Work out the finished part from the listing and answer in its coordinate system (mm). Give positions to 0.01 mm unless a question says otherwise; leave off trailing zeros. Write each loop counter-clockwise with the first axis right and the second up, starting at its lowest first coordinate (ties: lowest second). Pieces come first, ordered by that corner, then holes.
1) Find section B-B (y = 132.5). Determine the outline of the cut face in (x, z).
2) Find section D-D (x = 178.5). Determine the outline of the cut face in (y, z).
3) Straight lines are drawn through the part: probe 1 along X at (y, z) = (11, 1.5); probe 2 along Z at (x, y) = (-214.5, 116); probe 3 along X at (y, z) = (8, 2.75). For each, find the intervals that lie inside material, in ascending order.
4) Find section C-C (y = -32.5). Count the separate pieces of the cut face and the enclosed holes in it, plus the area to 3 significant figures.
5) Determine the mould class of faces 1 (the face through (-174.115, -38.296, 3.042)), 2 (the face through (-2.62, -41.8, 3.04)), 3 (the face through (-203, -32, 8)) for opening direction Y: pulls with the +Y half, pulls with the -Y half, needs draft (parallel to the pull), parting line crosses it, or undercut.
6) Given pin 1 Ø0.6 at (y, z) = (-25.5, 6.5) entering from -X; pin 2 Ø0.6 at (y, z) = (5.5, 6.5) entering from +X; pin 3 Ø0.6 at (x, z) = (-120, 6.5) entering from -Y, each flat-ended and moving along its own axis, determine where each tip first touches the part or whether it passes through.
7) Find section A-A (x = -204). Determine the outline of the cut face in (y, z), plus the area to 3 significant figures.
```python
from build123d import *

# Parameters (mm, degrees)
ESBO_O1_W                 = 485
ESBO_O1_H                 = 450
RESSALTO_EXTRUS_O1_DEPTH  = 6
ESBO_O2_W                 = 39.943598922
ESBO_O2_H                 = 30
RESSALTO_EXTRUS_O2_DEPTH  = 2
PADR_O_LINEAR1_COUNT      = 4
PADR_O_LINEAR1_PITCH      = 83
PADR_O_LINEAR1_COUNT_DIR2 = 2
PADR_O_LINEAR1_PITCH_DIR2 = 40
ESBO_O3_R                 = 9.525
CORTE_EXTRUS_O1_DEPTH     = 331.858353378
PADR_O_LINEAR2_COUNT      = 4
PADR_O_LINEAR2_PITCH      = 83
PADR_O_LINEAR2_COUNT_DIR2 = 2
PADR_O_LINEAR2_PITCH_DIR2 = 40
CHANFRO1_SIZE             = 2
CHANFRO1_SIZE2            = 3.464101615


with BuildPart() as part:
    # Esboço1 → Ressalto-extrusão1 (new body)
    with BuildSketch(Plane.XY):
        Rectangle(ESBO_O1_W, ESBO_O1_H)
    extrude(amount=RESSALTO_EXTRUS_O1_DEPTH)

    # Esboço2 → Ressalto-extrusão2 (add)
    with BuildSketch(Plane.XY.offset(6)):
        with Locations((-202.528200539, 7.5)):
            Rectangle(ESBO_O2_W, ESBO_O2_H)
    ressalto_extrus_o2 = extrude(amount=RESSALTO_EXTRUS_O2_DEPTH)

    # Padrão linear1: Ressalto-extrus_o2 4 × 2
    with Locations(*[(i * PADR_O_LINEAR1_PITCH, -j * PADR_O_LINEAR1_PITCH_DIR2, 0) for i in range(PADR_O_LINEAR1_COUNT) for j in range(PADR_O_LINEAR1_COUNT_DIR2) if (i, j) != (0, 0)]):
        add(ressalto_extrus_o2)

    # Esboço3 → Corte-extrusão1 (cut, through all)
    with BuildSketch(Plane.XY.offset(6)):
        with Locations((-166.556401078, 7.5)):
            Circle(ESBO_O3_R)
    corte_extrus_o1 = extrude(amount=-CORTE_EXTRUS_O1_DEPTH, mode=Mode.SUBTRACT)

    # Padrão linear2: Corte-extrus_o1 4 × 2
    with Locations(*[(i * PADR_O_LINEAR2_PITCH, -j * PADR_O_LINEAR2_PITCH_DIR2, 0) for i in range(PADR_O_LINEAR2_COUNT) for j in range(PADR_O_LINEAR2_COUNT_DIR2) if (i, j) != (0, 0)]):
        add(corte_extrus_o1, mode=Mode.SUBTRACT)

    # Chanfro1
    chanfro1_edges = [part.edges().sort_by_distance(p)[0] for p in [
        (0, 225, 0),
        (242.5, 0, 0),
        (0, -225, 0),
        (-242.5, 0, 0),
    ]]
    chanfro1_side = [part.faces().sort_by_distance(p)[0] for p in [
        (0, -218.383921101, 0),
    ]]
    chamfer(chanfro1_edges, length=CHANFRO1_SIZE, length2=CHANFRO1_SIZE2, reference=chanfro1_side[0])


solid = part.part
```
Results:
1. outline: (-242.5, 3.46) - (-240.5, 0) - (240.5, 0) - (242.5, 3.46) - (242.5, 6) - (-242.5, 6) - close
2. outline: (-225, 3.46) - (-223, 0) - (223, 0) - (225, 3.46) - (225, 6) - (-225, 6) - close
3. probe 1: x = -241.37 to -175.42, -157.7 to -92.42, -74.7 to -9.42, 8.3 to 73.58, 91.3 to 241.37
3. probe 2: z = 0 to 6
3. probe 3: x = -242.09 to -176.07, -157.04 to -93.07, -74.04 to -10.07, 8.96 to 72.93, 91.96 to 242.09
4. separate pieces: 5
4. enclosed holes: 0
4. area: 2,770 mm2
5. face 1: undercut
5. face 2: undercut
5. face 3: needs draft
6. pin 1: stops at x = -222.5
6. pin 2: stops at x = 66.44
6. pin 3: stops at y = -47.5
7. outline: (-225, 3.46) - (-223, 0) - (223, 0) - (225, 3.46) - (225, 6) - (22.5, 6) - (22.5, 8) - (-7.5, 8) - (-7.5, 6) - (-17.5, 6) - (-17.5, 8) - (-47.5, 8) - (-47.5, 6) - (-225, 6) - close
7. area: 2,810 mm2
